Here's how the part is built. I have some questions about the finished solid (model axes, mm). Face numbers are marked on the shaded views. A direction names the side the tool comes from. Round coordinates to 2 decimals unless told otherwise and drop trailing zeros. Loops run counter-clockwise (first coordinate to the right, second up) from the corner with the lowest first, then second, coordinate; pieces in that order, holes last. Notation, with made-up numbers: M -14.5,4.25 L 17.5,4.25 A32 ccw 17.5,40.25 Z; hole C -17,52 d2. An arc over 180 degrees is marked long. Write each question's results on one line, items separated by ' | '. Start each with the question number.
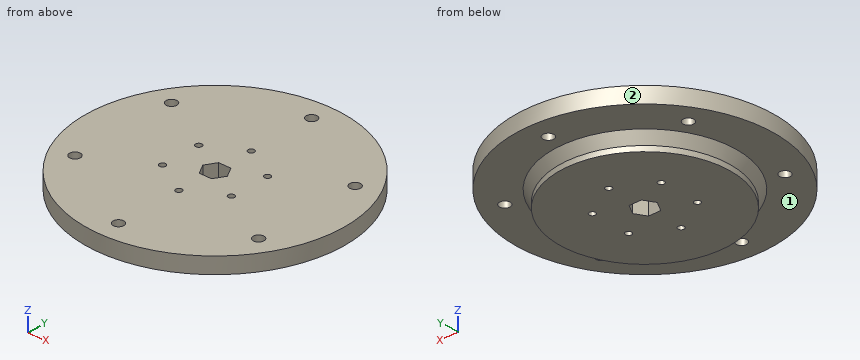
Autodesk Inventor part; units mm, degrees
ref_plane "YZ Plane" through (0, 0, 0) normal (1, 0, 0) x (0, 1, 0)
ref_plane "XZ Plane" through (0, 0, 0) normal (0, 1, 0) x (-1, 0, 0)
ref_plane "XY Plane" through (0, 0, 0) normal (0, 0, 1) x (1, 0, 0)
sketch "Sketch1" plane through (0, 0, 0) normal (0, 0, 1) x (1, 0, 0)
  circle A0 centre (0, 0) radius 76.2
  dimension "d0" = 152.4
extrude "Extrusion1" add sketch "Sketch1" along normal blind 9.525
sketch "Sketch9" plane through (0, 0, 9.525) normal (0, 0, 1) x (1, 0, 0)
  circle A0 centre (0, 0) radius 76.2
  point P0 (0, 63.5)
  point P1 (-54.9926, 31.75)
  point P2 (-54.9926, -31.75)
  point P3 (0, -63.5)
  point P4 (54.9926, -31.75)
  point P5 (54.9926, 31.75)
  dimension "d47" = 63.5
  dimension "d50" = 360
hole "Wheel Mount Holes" at (0, 63.5, 9.525) at (-54.9926, 31.75, 9.525) at (-54.9926, -31.75, 9.525) at (0, -63.5, 9.525) at (54.9926, -31.75, 9.525) at (54.9926, 31.75, 9.525) direction (0, 0, -1) diameter 6.4008 end through all
sketch "Sketch6" plane through (0, 0, 0) normal (0, 0, -1) x (-1, 0, 0)
  circle A0 centre (0, 0) radius 76.2
  circle A1 centre (0, 0) radius 53.975
  dimension "d59" = 107.95
extrude "Extrusion4" add sketch "Sketch6" along normal blind 6.35 draft -30 contours A1
sketch "Sketch10" plane through (0, 0, -6.35) normal (0, 0, -1) x (-1, 0, 0)
  circle A0 centre (0, 0) radius 50.3088
extrude "Extrusion6" add sketch "Sketch10" along normal blind 3.175
sketch "Sketch11" plane through (0, 0, -9.525) normal (0, 0, -1) x (-1, 0, 0)
  circle A0 centre (0, 0) radius 50.3088
  point P0 (0, 23.8125)
  point P1 (-20.6222, 11.9063)
  point P2 (-20.6222, -11.9062)
  point P3 (0, -23.8125)
  point P4 (20.6222, -11.9063)
  point P5 (20.6222, 11.9062)
  dimension "d62" = 23.8125
  dimension "d65" = 360
hole "Sprocket Mount Holes" at (0, 23.8125, -9.525) at (20.6222, 11.9063, -9.525) at (20.6222, -11.9062, -9.525) at (0, -23.8125, -9.525) at (-20.6222, -11.9063, -9.525) at (-20.6222, 11.9062, -9.525) direction (0, 0, 1) diameter 3.683 end through all
sketch "Sketch12" plane through (0, 0, 9.525) normal (0, 0, 1) x (1, 0, 0)
  circle A0 centre (0, 0) radius 76.2
  line L0 (3.6808, 6.3754) -> (7.3617, 0)
  line L1 (7.3617, 0) -> (3.6808, -6.3754)
  line L2 (3.6808, -6.3754) -> (-3.6808, -6.3754)
  line L3 (-3.6808, -6.3754) -> (-7.3617, 0)
  line L4 (-7.3617, 0) -> (-3.6808, 6.3754)
  line L5 (-3.6808, 6.3754) -> (3.6808, 6.3754)
  point P0 (0, 6.3754)
  dimension "d74" = 12.7508
extrude "Hex Bore" cut sketch "Sketch12" against normal through all contours L0 L1 L2 L3 L4 L5
properties part number "hub"
Item 1: I'm going to push flat-ended pins straight in: pin 1 (8 mm diameter, centred on y = -4, z = -2.5, fed in from +X); pin 2 (10 mm diameter, centred on x = 54.99, y = 31.75, fed in from -Z); pin 3 (10 mm diameter, centred on y = 52.5, z = 5, fed in from +X). Where does each tip first touch, or does it pass through?
Item 2: Which directions (+Z, -Z, +X, -X, +Y, -Y) give clear straight access to the entire face, cutting with the end or side of a thin tool? Please do the marked faces 1 and 2.
Item 3: I need wall thicknesses on L1, parallel to Y at x = 0, z = 6.25; L2, parallel to Z at x = -46, y = 49.5 (3 decimals); L3, parallel to Y at x = 55.5, z = 3.25. Which ranges of each line are inside material? Lowest first, please.
Item 4: If we section it at A-A on x = 0: Count the separate pieces of the cut face and the enclosed holes in it, and give its area (3 significant figures).
Item 5: If we section it at C-C on y = -63.5: Please give me the cut outline in (x, z) (3 decimals).
Numbers:
1) pin 1: x = 76.19 | pin 2: z = 0 | pin 3: x = 59.58
2) face 1: -Z | face 2: +Z, -Z
3) L1: -76.2 to -66.7, -60.3 to -25.65, -21.97 to -6.38, 6.38 to 21.97, 25.65 to 60.3, 66.7 to 76.2 | L2: 0 to 9.525 | L3: -52.21 to -34.91, -28.59 to 28.59, 34.91 to 52.21
4) separate pieces: 6 | enclosed holes: 0 | area: 1,930 mm²
5) outline: M -42.121,0 L -3.2,0 L -3.2,9.525 L -42.121,9.525 Z; M 3.2,0 L 42.121,0 L 42.121,9.525 L 3.2,9.525 Z
